```python
from build123d import *

# Parameters (mm, degrees)
F0_W           = 6.3491229296
F0_H           = 12.7
F1_DEPTH       = 3.175
F2_W           = 6.3491229296
F2_H           = 12.7
F3_DEPTH       = 6.35
F5_D           = 3.175
F5_CBORE_D     = 5.715
F5_CBORE_DEPTH = 1.905
F6_SIZE        = 3.175
F7_SIZE        = 1.5875
F8_SIZE        = 1.5875
F9_SIZE        = 1.5875
F10_SIZE       = 1.5875


with BuildPart() as f1:
    # F0 (on Top) → F1 (new body)
    with BuildSketch(Plane.XY):
        with Locations((15.8745614648, -6.35)):
            Rectangle(F0_W, F0_H)
        Polygon((12.7, 0), (12.7, 12.7), (-12.7, 12.7), (-12.7, -12.7), (12.7, -12.7), align=None)
    extrude(amount=-F1_DEPTH)

    # F2 (on face) → F3 (join)
    with BuildSketch(Plane(origin=(0, 0, -3.175), x_dir=(1, 0, 0), z_dir=(0, 0, -1))):
        with Locations((15.8745614648, 6.35)):
            Rectangle(F2_W, F2_H)
    extrude(amount=F3_DEPTH)

    # F5 (through all)
    with Locations(Plane.XY):
        with Locations((0, 0)):
            CounterBoreHole(F5_D / 2, F5_CBORE_D / 2, F5_CBORE_DEPTH)

    # F6
    f6_edges = [f1.edges().sort_by_distance(p)[0] for p in [
        (12.7, 12.7, -1.5875),
    ]]
    chamfer(f6_edges, length=F6_SIZE)

    # F7
    f7_edges = [f1.edges().sort_by_distance(p)[0] for p in [
        (19.049123, 0, -4.7625),
    ]]
    chamfer(f7_edges, length=F7_SIZE)

    # F8
    f8_edges = [f1.edges().sort_by_distance(p)[0] for p in [
        (19.049123, -12.7, -4.7625),
    ]]
    chamfer(f8_edges, length=F8_SIZE)

    # F9
    f9_edges = [f1.edges().sort_by_distance(p)[0] for p in [
        (12.7, 0, -6.35),
    ]]
    chamfer(f9_edges, length=F9_SIZE)

    # F10
    f10_edges = [f1.edges().sort_by_distance(p)[0] for p in [
        (12.7, -12.7, -6.35),
    ]]
    chamfer(f10_edges, length=F10_SIZE)


solid = f1.part
```
Input: part model. Units: mm. Frame: model coordinates. A direction names the side the tool comes from. Give positions to 0.01 mm unless a question says otherwise; leave off trailing zeros. Order: outer loops, then holes, each group sorted by start corner. A loop starts at its lowest first (then second) coordinate and runs counter-clockwise, first axis right, second up. Notation, with made-up numbers: M 83,54 L 100,54 A25 cw 100,89 Z; hole C 79,52.5 d1. An arc over 180 degrees is marked long. Return JSON: item names as keys, results as strings.
1) Contact query for flat-ended pins moving along their axis: pin 1 (5 mm diameter, centred on x = 0, y = 0, fed in from -Z) (3 decimals); pin 2 (3 mm diameter, centred on y = 0, z = -8.5, fed in from -X); pin 3 (1.4 mm diameter, centred on x = 15, z = -3.5, fed in from +Y); pin 4 (1.5 mm diameter, centred on x = 12.5, y = -2.5, fed in from -Z) (3 decimals). Output: stop coordinate, or through.
Taken from the geometry:
{"pin 1": "stops at z = -3.175", "pin 2": "stops at x = 12.79", "pin 3": "stops at y = 0", "pin 4": "stops at z = -9.525"}
2) Line query: L1, parallel to Y at x = 0, z = -1.25; L2, parallel to Y at x = 0, z = -2.55; L3, parallel to Z at x = -1, y = -10.25 (3 decimals). Output: solid intervals per line, ascending. Write a range as [from, to].
Taken from the geometry:
{"L1": "y = [-12.7, -2.86], [2.86, 12.7]", "L2": "y = [-12.7, -1.59], [1.59, 12.7]", "L3": "z = [-3.175, 0]"}
3) Section query A-A on x = 0. Output: boundary loops of the cut face in (y, z) (1 decimal), and give its area (3 significant figures).
Taken from the geometry:
{"outline": "M -12.7,-3.2 L -1.6,-3.2 L -1.6,-1.9 L -2.9,-1.9 L -2.9,0 L -12.7,0 Z; M 1.6,-3.2 L 12.7,-3.2 L 12.7,0 L 2.9,0 L 2.9,-1.9 L 1.6,-1.9 Z", "area": "65.7 mm2"}
4) Section query C-C on y = -8. Output: boundary loops of the cut face in (x, z) (3 decimals), and give its area (3 significant figures).
Taken from the geometry:
{"outline": "M -12.7,-3.175 L 12.7,-3.175 L 12.7,-9.525 L 19.049,-9.525 L 19.049,0 L -12.7,0 Z", "area": "141 mm2"}
5) Section query B-B on z = -7.5. Output: boundary loops of the cut face in (x, y), and give its area (3 significant figures).
Taken from the geometry:
{"outline": "M 12.7,-11.11 L 14.29,-12.7 L 17.46,-12.7 L 19.05,-11.11 L 19.05,-1.59 L 17.46,0 L 14.29,0 L 12.7,-1.59 Z", "area": "75.6 mm2"}
6) Section query D-D on x = 5.5. Output: boundary loops of the cut face in (y, z) (3 decimals).
Taken from the geometry:
{"outline": "M -12.7,-3.175 L 12.7,-3.175 L 12.7,0 L -12.7,0 Z"}
7) Mould query, pull axis Y, two halves, no side actions, for faces 1 (the face through (16, -6, -9.525)), 2 (the face through (0.34, -1.55, -2.55)), 3 (the face through (13.483, -0.805, -6.306)), 4 (the face through (6, -12.7, -3)). Classes: released by +Y, released by -Y, zero draft, split by the parting line, or undercut.
Taken from the geometry:
{"face 1": "zero draft", "face 2": "undercut", "face 3": "released by +Y", "face 4": "released by -Y"}
8) Access query for faces 5 (the face through (13.505, -11.917, -6.306)), 6 (the face through (12.7, -6, -6)), 7 (the face through (2.726, 0.858, -0.939)), 8 (the face through (12.7, 5, -2)). Directions: +Z, -Z, +X, -X, +Y, -Y. A direction counts if a zero-diameter tool reaches every point of the face in a straight line with its end or side. Return the directions, or none.
Taken from the geometry:
{"face 5": "-Z, -X, -Y", "face 6": "-Z, -X, +Y, -Y", "face 7": "+Z", "face 8": "+Z, -Z, +X, +Y"}
